```python
from build123d import *

# Parameters (mm, degrees)
CROQUIS1_W              = 212.725
CROQUIS1_H              = 187.325
CROQUIS1_W_2            = 203.2
CROQUIS1_H_2            = 177.8
SALIENTE_EXTRUIR1_DEPTH = 63.607999784
VACIADO1_T              = -4.7625
CROQUIS2_W              = 20
CROQUIS2_H              = 5.08
CROQUIS2_W_2            = 5.08
CROQUIS2_H_2            = 20
SALIENTE_EXTRUIR3_DEPTH = 25.4
CROQUIS2_5_W            = 5.08
CROQUIS2_5_H            = 20
CROQUIS2_5_W_2          = 20
CROQUIS2_5_H_2          = 5.08
SALIENTE_EXTRUIR4_DEPTH = 6.5
CROQUIS3_W              = 94.9325
CROQUIS3_H              = 63.1825
CORTAR_EXTRUIR1_DEPTH   = 156.343564234
SALIENTE_EXTRUIR5_DEPTH = 63.607999784
CROQUIS5_W              = 122.555
CROQUIS5_H              = 30.1625
CORTAR_EXTRUIR2_DEPTH   = 156.343564234
CROQUIS6_W              = 122.555
CROQUIS6_H              = 4.7625
SALIENTE_EXTRUIR6_DEPTH = 63.607999784
CROQUIS7_W              = 154.94
CROQUIS7_H              = 82.660152575
CORTAR_EXTRUIR3_DEPTH   = 58.845499784


with BuildPart() as part:
    # Croquis1 → Saliente-Extruir1 (new body)
    # profile 1 of 2: a face of its own
    with BuildSketch(Plane(origin=(0, 0, 0), x_dir=(1, 0, 0), z_dir=(0, 1, 0))):
        Rectangle(CROQUIS1_W, CROQUIS1_H)
        Rectangle(CROQUIS1_W_2, CROQUIS1_H_2, mode=Mode.SUBTRACT)
    # profile 2 of 2: a face of its own
    with BuildSketch(Plane(origin=(0, 0, 0), x_dir=(1, 0, 0), z_dir=(0, 1, 0))):
        Rectangle(CROQUIS1_W_2, CROQUIS1_H_2)
    extrude(amount=SALIENTE_EXTRUIR1_DEPTH)

    # Vaciado1
    vaciado1_openings = [part.faces().sort_by_distance(p)[0] for p in [
        (0, 63.607999784, 0),
    ]]
    offset(amount=VACIADO1_T, openings=vaciado1_openings, kind=Kind.INTERSECTION)

    # Croquis2 → Saliente-Extruir3 (add)
    with BuildSketch(Plane(origin=(0, 4.7625, 0), x_dir=(1, 0, 0), z_dir=(0, 1, 0))):
        with Locations((-44.45, 66.04)):
            Rectangle(CROQUIS2_W, CROQUIS2_H)
        with Locations((-80.01, 0)):
            Rectangle(CROQUIS2_W_2, CROQUIS2_H_2)
        with Locations((0, -67.31)):
            Rectangle(CROQUIS2_W, CROQUIS2_H)
        with Locations((80.01, -28.575)):
            Rectangle(CROQUIS2_W_2, CROQUIS2_H_2)
    extrude(amount=SALIENTE_EXTRUIR3_DEPTH)

    # Croquis2<5> → Saliente-Extruir4 (add)
    with BuildSketch(Plane(origin=(0, 4.7625, 0), x_dir=(1, 0, 0), z_dir=(0, 1, 0))):
        with Locations((-74.93, 0)):
            Rectangle(CROQUIS2_5_W, CROQUIS2_5_H)
        with Locations((0, -62.23)):
            Rectangle(CROQUIS2_5_W_2, CROQUIS2_5_H_2)
        with Locations((74.93, -28.575)):
            Rectangle(CROQUIS2_5_W, CROQUIS2_5_H)
    extrude(amount=SALIENTE_EXTRUIR4_DEPTH)

    # Croquis3 → Cortar-Extruir1 (cut, through all)
    with BuildSketch(Plane(origin=(0, 63.607999784, 0), x_dir=(1, 0, 0), z_dir=(0, 1, 0))):
        with Locations((58.89625, 62.07125)):
            Rectangle(CROQUIS3_W, CROQUIS3_H)
    extrude(amount=-CORTAR_EXTRUIR1_DEPTH, mode=Mode.SUBTRACT)

    # Croquis4 → Saliente-Extruir5 (add)
    with BuildSketch(Plane(origin=(0, 0, 0), x_dir=(1, 0, 0), z_dir=(0, 1, 0))):
        Polygon((11.43, 93.6625), (16.1925, 93.6625), (16.1925, 35.2425), (106.3625, 35.2425), (106.3625, 30.48), (11.43, 30.48), align=None)
    extrude(amount=SALIENTE_EXTRUIR5_DEPTH)

    # Croquis5 → Cortar-Extruir2 (cut, through all)
    with BuildSketch(Plane(origin=(0, 0, 0), x_dir=(1, 0, 0), z_dir=(0, 1, 0))):
        with Locations((-45.085, 78.58125)):
            Rectangle(CROQUIS5_W, CROQUIS5_H)
    extrude(amount=CORTAR_EXTRUIR2_DEPTH, mode=Mode.SUBTRACT)

    # Croquis6 → Saliente-Extruir6 (add)
    with BuildSketch(Plane(origin=(0, 0, 0), x_dir=(1, 0, 0), z_dir=(0, 1, 0))):
        with Locations((-45.085, 65.88125)):
            Rectangle(CROQUIS6_W, CROQUIS6_H)
    extrude(amount=SALIENTE_EXTRUIR6_DEPTH)

    # Croquis7 → Cortar-Extruir3 (cut)
    with BuildSketch(Plane(origin=(0, 63.607999784, 0), x_dir=(1, 0, 0), z_dir=(0, 1, 0))):
        with Locations((0, -23.439923713)):
            Rectangle(CROQUIS7_W, CROQUIS7_H)
    extrude(amount=-CORTAR_EXTRUIR3_DEPTH, mode=Mode.SUBTRACT)


solid = part.part
```
Check sheet for the modelled part. Datum: model origin and axes. Units: mm. A direction names the side the tool comes from. Give positions to 0.01 mm unless a question says otherwise; leave off trailing zeros. Write each loop counter-clockwise with the first axis right and the second up, starting at its lowest first coordinate (ties: lowest second). Pieces come first, ordered by that corner, then holes.
Item 1: Draft check along X on faces 3 (the face through (61, 31, -35.242)), 4 (the face through (106.362, 31, 28)), 5 (the face through (-80, 30.162, 0)). Enter one of: released by +X, released by -X, zero draft, split by the parting line, or undercut.
Item 2: Cross-section at A-A (y = 20). Count the separate pieces of the cut face and the enclosed holes in it, and give its area (3 significant figures).
Item 3: Scan lines: L1, parallel to X at y = 17, z = 67; L2, parallel to X at y = 28.5, z = 9.5; L3, parallel to X at y = 41, z = 64.5. Record each from-to range of solid material in increasing order.
Item 4: Access from +Z, -Z, +X, -X, +Y, -Y to the whole of each face (thin tool, end or side, straight path). Record for faces 1 (the face through (57, 34, -30.48)), 2 (the face through (-106.363, 31, 14)).
Item 5: Cross-section at D-D (y = 57). Enter the section's corners in (x, z).
Item 6: Gauge pin test, flat ends, axial feed: pin 1 (3 mm diameter, centred on x = 40, y = 41.5, fed in from -Z); pin 2 (4 mm diameter, centred on x = 81, z = 30, fed in from +Y); pin 3 (2 mm diameter, centred on x = -25.5, z = 59, fed in from +Y). Record the tip position at first contact, or that the pin passes through.
Item 7: Cross-section at B-B (x = -69.5). Enter the section's corners in (y, z), and give its area (3 significant figures).
Item 8: Cross-section at C-C (z = -37.5). Enter the section's corners in (x, y), and give its area (3 significant figures).
Report:
1. face 3: zero draft
1. face 4: released by +X
1. face 5: undercut
2. separate pieces: 4
2. enclosed holes: 1
2. area: 3,780 mm2
3. L1: x = -106.36 to -101.6, -10 to 10, 101.6 to 106.36
3. L2: x = -106.36 to -101.6, -82.55 to -77.47, 101.6 to 106.36
3. L3: x = -106.36 to -101.6, 101.6 to 106.36
4. face 1: +Y
4. face 2: +Z, -Z, -X, +Y, -Y
5. outline: (-106.36, -68.26) - (16.19, -68.26) - (16.19, -35.24) - (106.36, -35.24) - (106.36, 93.66) - (-106.36, 93.66) - close; hole (-101.6, -63.5) - (11.43, -63.5) - (11.43, -30.48) - (101.6, -30.48) - (101.6, 88.9) - (-101.6, 88.9) - close
6. pin 1: stops at z = -35.24
6. pin 2: stops at y = 30.16
6. pin 3: stops at y = 4.76
7. outline: (0, -68.26) - (63.61, -68.26) - (63.61, -63.5) - (4.76, -63.5) - (4.76, 88.9) - (63.61, 88.9) - (63.61, 93.66) - (0, 93.66) - close
7. area: 1,330 mm2
8. outline: (-106.36, 0) - (16.19, 0) - (16.19, 63.61) - (11.43, 63.61) - (11.43, 4.76) - (-101.6, 4.76) - (-101.6, 63.61) - (-106.36, 63.61) - close
8. area: 1,140 mm2
